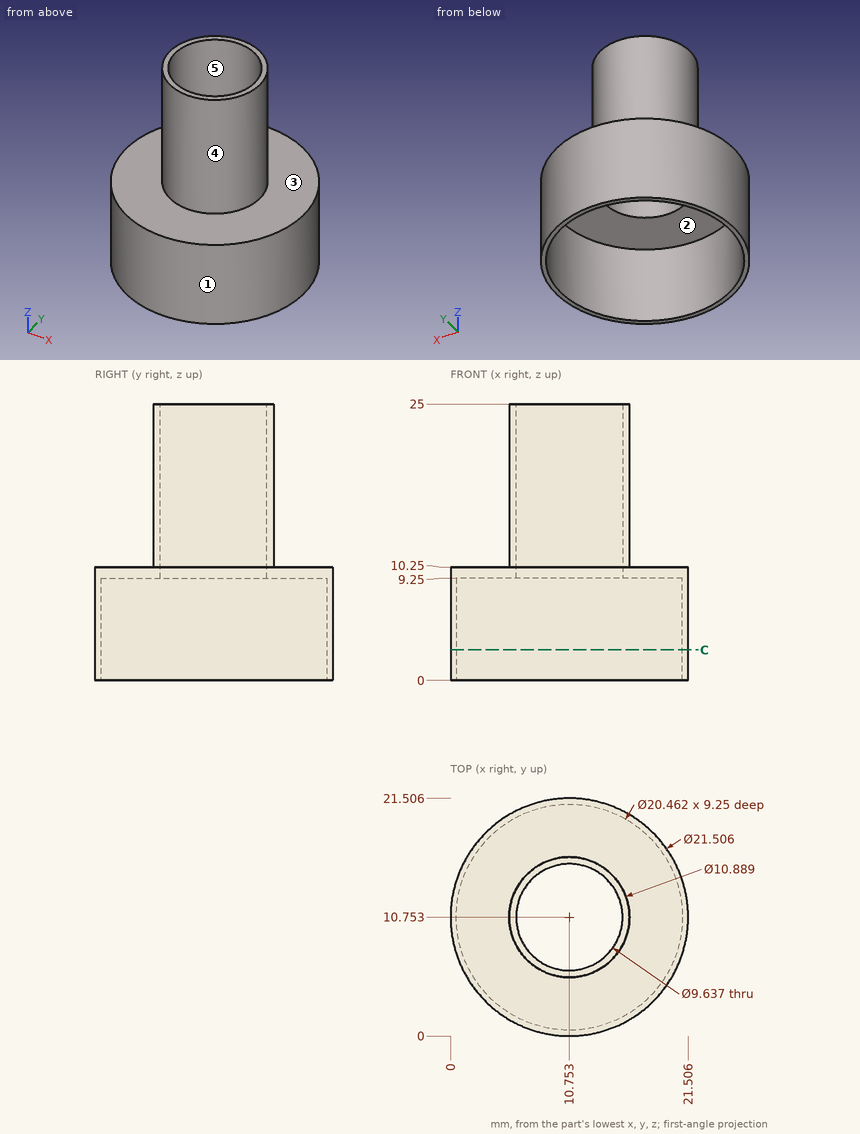
Here's the drawing with two shaded views (mm, measured from the low corner). I have some questions. A direction names the side the tool comes from. Coordinates: 2 decimals unless noted, no trailing zeros. Write each loop counter-clockwise with the first axis right and the second up, starting at its lowest first coordinate (ties: lowest second). Pieces come first, ordered by that corner, then holes.
Item 1: If I drill on line 1 (X direction, y = 10.5, z = 12.75) (1 decimal); line 2 (Z direction, x = 9.5, y = 19.75), over which ranges is the centre line in solid material (lowest first)?
Item 2: Will these pins go through, and if not, where does the flat tip stop? pin 1 (10 mm diameter, centred on x = 13.5, z = 9.5, fed in from -Y); pin 2 (1 mm diameter, centred on x = 16, z = 16, fed in from -Y) (1 decimal); pin 3 (7.5 mm diameter, centred on x = 10.75, y = 10.75, fed in from +Z); pin 4 (8 mm diameter, centred on x = 17.5, z = 10, fed in from +Y).
Item 3: If we mould it in two halves opening along Y, with no side actions, what happens to the marked faces 3, 4 and 5? For each: +Y half, -Y half, draft (parallel to the pull), parting line (faces both ways), or undercut.
Item 4: On a 3-axis mill with a long thin cutter (end or side, diameter ignored), from which of +Z, -Z, +X, -X, +Y, -Y can I reach the whole of each face in a straight line? I mean the marked faces 1 and 2. Say none if no direction works.
Item 5: I want a section at C-C on z = 2.75. Write out the boundary of the cut face in (x, y) (1 decimal).
Findings below:
1. line 1: x = 5.3 to 5.9, 15.6 to 16.2
1. line 2: z = 9.25 to 10.25
2. pin 1: stops at y = 0
2. pin 2: stops at y = 8.1
2. pin 3: passes through
2. pin 4: stops at y = 21.15
3. face 3: draft
3. face 4: parting line
3. face 5: undercut
4. face 1: +Z, -Z
4. face 2: -Z
5. outline: circle Ø21.5 at (10.8, 10.8); hole circle Ø20.5 at (10.8, 10.8)
